Verification items for the finished model (mm, model axes). Give positions to 0.01 mm unless a question says otherwise; leave off trailing zeros. Loops run counter-clockwise (first coordinate to the right, second up) from the corner with the lowest first, then second, coordinate; pieces in that order, holes last. Notation, with made-up numbers: M 14.25,27.25 L 42.25,27.25 A20 ccw 42.25,45.25 Z; hole C 37.5,-12 d3. An arc over 180 degrees is marked long. Answer in a Markdown table with one row per item.
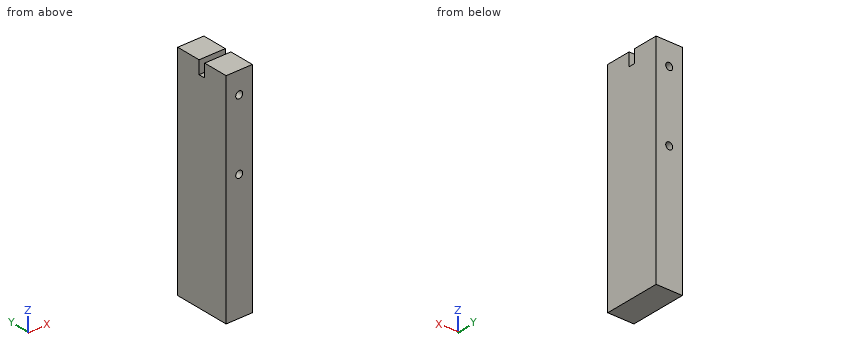
```python
from build123d import *

# Parameters (mm, degrees)
SKETCH1_W          = 12
SKETCH1_H          = 100
SKETCH1_R          = 1.6
EXTRUDE1_DEPTH     = 13
SKETCH2_W          = 12
SKETCH2_H          = 6
CUT_EXTRUDE1_DEPTH = 1.5


with BuildPart() as part:
    # Sketch1 → Extrude1 (new body, symmetric)
    with BuildSketch(Plane(origin=(0, 0, 0), x_dir=(1, 0, 0), z_dir=(0, 1, 0))):
        with Locations((0, 50)):
            Rectangle(SKETCH1_W, SKETCH1_H)
        with Locations(Location((0, 10, 0), (0, 0, 270))):  # turned: the seam where the file's is
            Circle(SKETCH1_R, mode=Mode.SUBTRACT)
        with Locations(Location((0, 42, 0), (0, 0, 270))):  # turned: the seam where the file's is
            Circle(SKETCH1_R, mode=Mode.SUBTRACT)
    extrude(amount=EXTRUDE1_DEPTH, both=True)

    # Sketch2 → Cut-Extrude1 (cut, symmetric)
    with BuildSketch(Plane(origin=(0, 0, 0), x_dir=(1, 0, 0), z_dir=(0, 1, 0))):
        with Locations((0, 3)):
            Rectangle(SKETCH2_W, SKETCH2_H)
    extrude(amount=CUT_EXTRUDE1_DEPTH, both=True, mode=Mode.SUBTRACT)


solid = part.part
```
Item 1: Sectioned sample at B-B (z = -10). Record the cut outline in (x, y), and give its area (3 significant figures).
Reported:
| item | result |
|---|---|
| outline | M -6,-13 L -1.6,-13 L -1.6,13 L -6,13 Z; M 1.6,-13 L 6,-13 L 6,13 L 1.6,13 Z |
| area | 229 mm^2 |
Item 2: Scan lines: L1, parallel to X at y = -0.75, z = -10; L2, parallel to Z at x = 1.25, y = -1; L3, parallel to Z at x = -1, y = 3. Record each from-to range of solid material in increasing order. Write a range as [from, to].
Reported:
| item | result |
|---|---|
| L1 | x = [-6, -1.6], [1.6, 6] |
| L2 | z = [-100, -43], [-41, -11], [-9, -6] |
| L3 | z = [-100, -43.25], [-40.75, -11.25], [-8.75, 0] |
Item 3: Go/stop test with flat-tipped pins: pin 1 (4 mm diameter, centred on x = 4, y = -2.5, fed in from +Z); pin 2 (2.5 mm diameter, centred on x = 2.5, y = 0, fed in from +Z). Record where each tip stops, or that it passes through.
Reported:
| item | result |
|---|---|
| pin 1 | stops at z = 0 |
| pin 2 | stops at z = -6 |
Item 4: Sectioned sample at A-A (x = 0). Record the cut outline in (y, z).
Reported:
| item | result |
|---|---|
| outline | M -13,-100 L 13,-100 L 13,-43.6 L -13,-43.6 Z; M -13,-40.4 L 13,-40.4 L 13,-11.6 L -13,-11.6 Z; M -13,-8.4 L 13,-8.4 L 13,0 L 1.5,0 L 1.5,-6 L -1.5,-6 L -1.5,0 L -13,0 Z |
